Can you work these out from the drawing? Everything is in mm from the part's minimum corner. Round coordinates to 2 decimals unless told otherwise and drop trailing zeros. Loops run counter-clockwise (first coordinate to the right, second up) from the corner with the lowest first, then second, coordinate; pieces in that order, holes last. Notation, with made-up numbers: M 41,32 L 76,32 A29 ccw 76,58 Z; hole C 38,16 d6. An arc over 180 degrees is marked long. Use a Markdown table: item, result.
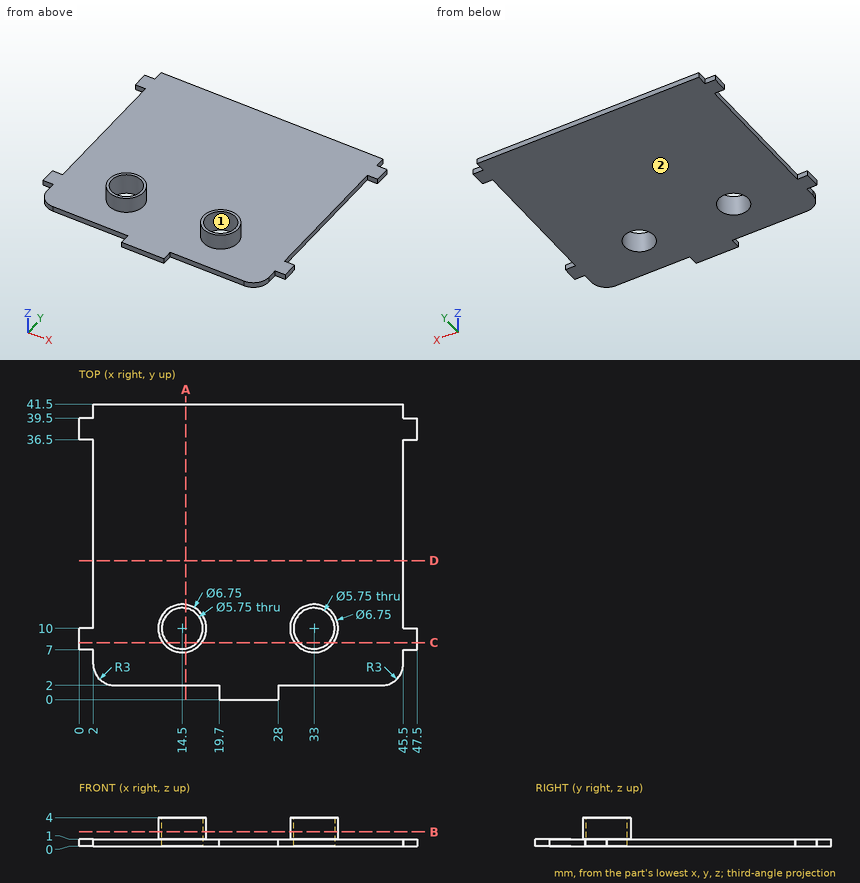
1. Imagine slicing it at A-A, the plane x = 15. Write out the boundary of the cut face in (y, z).
Answer sheet:
| item | result |
|---|---|
| outline | M 2,0 L 7.17,0 L 7.17,4 L 6.66,4 L 6.66,1 L 2,1 Z; M 12.83,0 L 41.5,0 L 41.5,1 L 13.34,1 L 13.34,4 L 12.83,4 Z |
2. Imagine slicing it at C-C, the plane y = 8. Write out the boundary of the cut face in (x, z) (1 decimal).
Answer sheet:
| item | result |
|---|---|
| outline | M 0,0 L 12.4,0 L 12.4,4 L 11.8,4 L 11.8,1 L 0,1 Z; M 16.6,0 L 30.9,0 L 30.9,4 L 30.3,4 L 30.3,1 L 17.2,1 L 17.2,4 L 16.6,4 Z; M 35.1,0 L 47.5,0 L 47.5,1 L 35.7,1 L 35.7,4 L 35.1,4 Z |
3. Imagine slicing it at B-B, the plane z = 2. State how many separate pieces and enclosed holes the cut face has.
Answer sheet:
| item | result |
|---|---|
| separate pieces | 2 |
| enclosed holes | 2 |
4. We'd pull the mould along X, two halves only. Please class the marked faces 1 and 2: +X half, -X half, draft (parallel to the pull), parting line (faces both ways), or undercut.
Answer sheet:
| item | result |
|---|---|
| face 1 | undercut |
| face 2 | draft |
5. Imagine slicing it at D-D, the plane y = 19.5. Write out the boundary of the cut face in (x, z).
Answer sheet:
| item | result |
|---|---|
| outline | M 2,0 L 45.5,0 L 45.5,1 L 2,1 Z |
6. For pin 1 Ø0.5 at (x, z) = (46.5, 0.5) entering from +Y; pin 2 Ø0.5 at (y, z) = (6, 0.5) entering from -X; pin 3 Ø0.5 at (y, z) = (1, 0.5) entering from -X, each with a flat end and sliding along its axis, tell me the tip position at first contact or that it passes through.
Answer sheet:
| item | result |
|---|---|
| pin 1 | y = 39.5 |
| pin 2 | x = 2 |
| pin 3 | x = 19.7 |
7. I need wall thicknesses on probe 1 along X at (y, z) = (11.5, 2.4) (1 decimal); probe 2 along X at (y, z) = (12.5, 1.1) (1 decimal); probe 3 along Z at (x, y) = (44, 28.5). Which ranges of each line are inside material? Lowest first, please. Write a range as from..to.
Answer sheet:
| item | result |
|---|---|
| probe 1 | 11.5..12, 17..17.5, 30..30.5, 35.5..36 |
| probe 2 | 12.2..13.1, 15.9..16.8, 30.7..31.6, 34.4..35.3 |
| probe 3 | 0..1 |
